Work out the finished part from the listing and answer in its coordinate system (mm). Face numbers are marked on the shaded views. A direction names the side the tool comes from. Round coordinates to 2 decimals unless told otherwise and drop trailing zeros. Loops run counter-clockwise (first coordinate to the right, second up) from the corner with the lowest first, then second, coordinate; pieces in that order, holes last. Notation, with made-up numbers: (52, -11) - (92, -11) arc R26 ccw to (92, 19) - close; hole circle Ø10 at (-14, -5). An arc over 180 degrees is marked (long way). Use CSV: the item, a comma, the result in double quotes. Start each with the question number.
from build123d import *

# Parameters (mm, degrees)
ESQUISSE2_R             = 2.5
ENL_V_MAT_EXTRU_1_DEPTH = 17
ENL_V_MAT_EXTRU_2_DEPTH = 8


with BuildPart() as part:
    # Esquisse1 → Révolution1 (revolve)
    with BuildSketch(Plane.XY):
        Polygon((0, 0), (0, 16), (8, 16), (8, 15), (6, 15), (6, 7), (8, 7), (8, 0), align=None)
    revolve(axis=Axis((0, 0, 0), (0, 1, 0)))

    # Esquisse2 → Enlèv. mat.-Extru.1 (cut, through all)
    with BuildSketch(Plane(origin=(0, 16, 0), x_dir=(1, 0, 0), z_dir=(0, 1, 0))):
        Circle(ESQUISSE2_R)
    extrude(amount=-ENL_V_MAT_EXTRU_1_DEPTH, mode=Mode.SUBTRACT)

    # Esquisse3 → Enlèv. mat.-Extru.2 (cut)
    with BuildSketch(Plane.XZ.offset(-15)):
        with BuildLine():
            ThreePointArc((5.981504002, -0.470754574), (5.528882211, 0), (5.981504002, 0.470754574))
            ThreePointArc((5.981504002, 0.470754574), (6, 0), (5.981504002, -0.470754574))
        make_face()
        with BuildLine():
            ThreePointArc((5.543277195, -2.296100594), (5.706339098, -1.854101966), (5.834219522, -1.400672183))
            ThreePointArc((5.834219522, -1.400672183), (5.258279454, -1.708518563), (5.543277195, -2.296100594))
        make_face()
        with BuildLine():
            ThreePointArc((4.562435794, -3.89668829), (4.472959669, -3.249795425), (5.115840986, -3.134991388))
            ThreePointArc((5.115840986, -3.134991388), (4.854101966, -3.526711514), (4.562435794, -3.89668829))
        make_face()
        with BuildLine():
            ThreePointArc((3.134991388, -5.115840986), (3.249795425, -4.472959669), (3.89668829, -4.562435794))
            ThreePointArc((3.89668829, -4.562435794), (3.526711514, -4.854101966), (3.134991388, -5.115840986))
        make_face()
        with BuildLine():
            ThreePointArc((1.400672183, -5.834219522), (1.708518563, -5.258279454), (2.296100594, -5.543277195))
            ThreePointArc((2.296100594, -5.543277195), (1.854101966, -5.706339098), (1.400672183, -5.834219522))
        make_face()
        with BuildLine():
            ThreePointArc((-0.470754574, -5.981504002), (0, -5.528882211), (0.470754574, -5.981504002))
            ThreePointArc((0.470754574, -5.981504002), (0, -6), (-0.470754574, -5.981504002))
        make_face()
        with BuildLine():
            ThreePointArc((-2.296100594, -5.543277195), (-1.708518563, -5.258279454), (-1.400672183, -5.834219522))
            ThreePointArc((-1.400672183, -5.834219522), (-1.854101966, -5.706339098), (-2.296100594, -5.543277195))
        make_face()
        with BuildLine():
            ThreePointArc((-3.89668829, -4.562435794), (-3.249795425, -4.472959669), (-3.134991388, -5.115840986))
            ThreePointArc((-3.134991388, -5.115840986), (-3.526711514, -4.854101966), (-3.89668829, -4.562435794))
        make_face()
        with BuildLine():
            ThreePointArc((-5.115840986, -3.134991388), (-4.472959669, -3.249795425), (-4.562435794, -3.89668829))
            ThreePointArc((-4.562435794, -3.89668829), (-4.854101966, -3.526711514), (-5.115840986, -3.134991388))
        make_face()
        with BuildLine():
            ThreePointArc((-5.834219522, -1.400672183), (-5.258279454, -1.708518563), (-5.543277195, -2.296100594))
            ThreePointArc((-5.543277195, -2.296100594), (-5.706339098, -1.854101966), (-5.834219522, -1.400672183))
        make_face()
        with BuildLine():
            ThreePointArc((-5.981504002, 0.470754574), (-5.528882211, 0), (-5.981504002, -0.470754574))
            ThreePointArc((-5.981504002, -0.470754574), (-6, 0), (-5.981504002, 0.470754574))
        make_face()
        with BuildLine():
            ThreePointArc((-5.543277195, 2.296100594), (-5.258279454, 1.708518563), (-5.834219522, 1.400672183))
            ThreePointArc((-5.834219522, 1.400672183), (-5.706339098, 1.854101966), (-5.543277195, 2.296100594))
        make_face()
        with BuildLine():
            ThreePointArc((-4.562435794, 3.89668829), (-4.472959669, 3.249795425), (-5.115840986, 3.134991388))
            ThreePointArc((-5.115840986, 3.134991388), (-4.854101966, 3.526711514), (-4.562435794, 3.89668829))
        make_face()
        with BuildLine():
            ThreePointArc((-3.134991388, 5.115840986), (-3.249795425, 4.472959669), (-3.89668829, 4.562435794))
            ThreePointArc((-3.89668829, 4.562435794), (-3.526711514, 4.854101966), (-3.134991388, 5.115840986))
        make_face()
        with BuildLine():
            ThreePointArc((-1.400672183, 5.834219522), (-1.708518563, 5.258279454), (-2.296100594, 5.543277195))
            ThreePointArc((-2.296100594, 5.543277195), (-1.854101966, 5.706339098), (-1.400672183, 5.834219522))
        make_face()
        with BuildLine():
            ThreePointArc((0.470754574, 5.981504002), (0, 5.528882211), (-0.470754574, 5.981504002))
            ThreePointArc((-0.470754574, 5.981504002), (0, 6), (0.470754574, 5.981504002))
        make_face()
        with BuildLine():
            ThreePointArc((2.296100594, 5.543277195), (1.708518563, 5.258279454), (1.400672183, 5.834219522))
            ThreePointArc((1.400672183, 5.834219522), (1.854101966, 5.706339098), (2.296100594, 5.543277195))
        make_face()
        with BuildLine():
            ThreePointArc((3.89668829, 4.562435794), (3.249795425, 4.472959669), (3.134991388, 5.115840986))
            ThreePointArc((3.134991388, 5.115840986), (3.526711514, 4.854101966), (3.89668829, 4.562435794))
        make_face()
        with BuildLine():
            ThreePointArc((5.115840986, 3.134991388), (4.472959669, 3.249795425), (4.562435794, 3.89668829))
            ThreePointArc((4.562435794, 3.89668829), (4.854101966, 3.526711514), (5.115840986, 3.134991388))
        make_face()
        with BuildLine():
            ThreePointArc((5.834219522, 1.400672183), (5.258279454, 1.708518563), (5.543277195, 2.296100594))
            ThreePointArc((5.543277195, 2.296100594), (5.706339098, 1.854101966), (5.834219522, 1.400672183))
        make_face()
    extrude(amount=ENL_V_MAT_EXTRU_2_DEPTH, mode=Mode.SUBTRACT)


solid = part.part
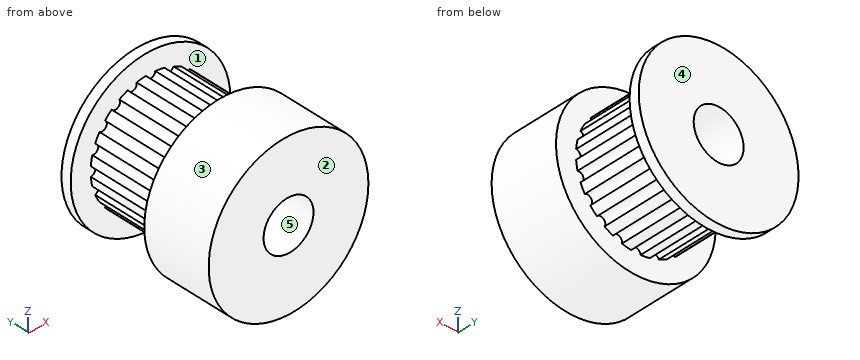
Item 1: The mould has two halves that part along Z. Classify the marked faces 3, 4 and 5: pulls with the +Z half, pulls with the -Z half, needs draft (parallel to the pull), parting line crosses it, or undercut.
Item 2: Which of the six approach directions +Z, -Z, +X, -X, +Y, -Y give full straight-line access (tool end or side, diameter ignored) to the marked faces 1 and 2?
Item 3: A cutting plane is placed at D-D (x = -3.5). Determine the outline of the cut face in (y, z).
Item 4: Each of these flat-tipped pins is pushed along its axis until it touches: pin 1 Ø6 at (y, z) = (10.5, -2) entering from +X; pin 2 Ø6 at (y, z) = (7, -5) entering from -X. Where does it stop, or does it pass through?
Item 5: A cutting plane is placed at B-B (z = 0). Determine the outline of the cut face in (x, y), plus the area to 3 significant figures.
Item 6: A cutting plane is placed at C-C (y = 2.5). Determine the outline of the cut face in (x, z).
Item 7: Find the intervals of material crossed by probe 1 along Y at (x, z) = (-7.5, 1.25); probe 2 along X at (y, z) = (11, 0), in increasing order. Write a range as [from, to].
Item 8: A cutting plane is placed at A-A (x = 0). Determine the outline of the cut face in (y, z).
Result sheet:
1,face 3,"parting line crosses it"
1,face 4,"needs draft"
1,face 5,"undercut"
2,face 1,"none"
2,face 2,"+Z, -Z, +X, -X, -Y"
3,outline,"(0, -7.19) - (7, -7.19) - (7, -4.38) - (15, -4.38) - (15, -7.19) - (16, -7.19) - (16, 7.19) - (15, 7.19) - (15, 4.38) - (7, 4.38) - (7, 7.19) - (0, 7.19) - close"
4,pin 1,"x = 5.98"
4,pin 2,"x = -7.75"
5,outline,"(-8, 0) - (-2.5, 0) - (-2.5, 16) - (-8, 16) - (-8, 15) - (-5.53, 15) - (-5.53, 7) - (-8, 7) - close; (2.5, 0) - (8, 0) - (8, 7) - (5.53, 7) - (5.53, 15) - (8, 15) - (8, 16) - (2.5, 16) - close"
5,area,"136 mm^2"
6,outline,"circle Ø16 at (0, 0); hole circle Ø5 at (0, 0)"
7,probe 1,"[0, 7], [15, 16]"
7,probe 2,"[-5.53, -2.5], [2.5, 5.53]"
8,outline,"(0, -8) - (7, -8) - (7, -5.53) - (15, -5.53) - (15, -8) - (16, -8) - (16, -2.5) - (0, -2.5) - close; (0, 2.5) - (16, 2.5) - (16, 8) - (15, 8) - (15, 5.53) - (7, 5.53) - (7, 8) - (0, 8) - close"
